For this review, take the finished solid that the model builds, in its own axes (mm). A direction names the side the tool comes from. Round coordinates to 2 decimals unless told otherwise and drop trailing zeros. Order: outer loops, then holes, each group sorted by start corner. A loop starts at its lowest first (then second) coordinate and runs counter-clockwise, first axis right, second up. Notation, with made-up numbers: M 42,7 L 65,7 A32 cw 65,43 Z; hole C 43,58.25 d5. An arc over 180 degrees is marked long. Put each result on its own line as item: value.
from build123d import *

# Parameters (mm, degrees)
F1_DEPTH = 15.24


with BuildPart() as f1:
    # F0 (on Front) → F1 (new body, symmetric)
    with BuildSketch(Plane.XZ):
        with BuildLine():
            ThreePointArc((39.819952, -34.683209), (43.15441, -51.434249), (51.5128, -66.328987))
            Line((51.5128, -66.328987), (81.9928, -66.328987))
            Line((81.9928, -66.328987), (64.616776, -18.092548))
            ThreePointArc((64.616776, -18.092548), (65.491758, -8.876663), (73.156603, -3.68549))
            Line((73.156603, -3.68549), (73.156603, 0))
            Line((73.156603, 0), (0, 0))
            Line((0, 0), (0, -7.535368))
            Line((0, -7.535368), (28.341651, -7.535368))
            Line((28.341651, -7.535368), (28.341651, -29.748611))
            Line((28.341651, -29.748611), (33.654915, -29.748611))
            ThreePointArc((33.654915, -29.748611), (37.603267, -31.134181), (39.819952, -34.683209))
        make_face()
    extrude(amount=F1_DEPTH, both=True)


solid = f1.part
(1) For faces 4 (the face through (73.157, 0, -2)), 5 (the face through (28.342, 0, -18)), 6 (the face through (73.426, -0.213, -42.548)), list the 3-axis set-ups (+Z, -Z, +X, -X, +Y, -Y) from which the entire face can be reached by the end or side of a thin tool; tool diameter is ignored.
A:
face 4: +Z, +X, +Y, -Y
face 5: -Z, -X, +Y, -Y
face 6: +X, +Y, -Y
(2) Add section A-A on x = 67. Give the boundary of the cut face in (y, z), then the cut area to 3 significant figures.
A:
outline: M -15.24,-66.33 L 15.24,-66.33 L 15.24,-24.71 L -15.24,-24.71 Z; M -15.24,-6.89 L 15.24,-6.89 L 15.24,0 L -15.24,0 Z
area: 1,480 mm2
(3) Add section B-B on y = -10. Give the boundary of the cut face in (x, z), then the cut area to 3 significant figures.
A:
outline: M 0,-7.54 L 28.34,-7.54 L 28.34,-29.75 L 33.65,-29.75 A6.32 cw 39.82,-34.68 A54.47 ccw 51.51,-66.33 L 81.99,-66.33 L 64.62,-18.09 A10.86 cw 73.16,-3.69 L 73.16,0 L 0,0 Z
area: 2,550 mm2
(4) To check wall thickness, follow L1, parallel to Z at x = 7, y = -9; L2, parallel to X at y = 9.5, z = -55.5; L3, parallel to Z at x = 32, y = -9. State the ranges of each line that lie inside material, in increasing order.
A:
L1: z = -7.54 to 0
L2: x = 44.85 to 78.09
L3: z = -29.75 to 0
(5) Draft analysis for pull direction Z (two halves, no side actions). For faces 1 (the face through (65.424, -0.213, -8.992)), 2 (the face through (67, 0, -66.329)), 3 (the face through (50, 15.24, -33)), state which applies: released by +Z, released by -Z, zero draft, split by the parting line, or undercut.
A:
face 1: undercut
face 2: released by -Z
face 3: zero draft
(6) Add section C-C on z = -47.5. Give the boundary of the cut face in (x, y), then the cut area to 3 significant figures.
A:
outline: M 41.87,-15.24 L 75.21,-15.24 L 75.21,15.24 L 41.87,15.24 Z
area: 1,020 mm2
(7) Add section D-D on x = 13. Give the boundary of the cut face in (y, z), then the cut area to 3 significant figures.
A:
outline: M -15.24,-7.54 L 15.24,-7.54 L 15.24,0 L -15.24,0 Z
area: 230 mm2
(8) Insertion check: pin 1 Ø14 at (x, y) = (11.5, -7.5) entering from -Z; pin 2 Ø1.8 at (y, z) = (5, -1) entering from +X; pin 3 Ø4.5 at (x, y) = (30, -3.5) entering from -Z. Each pin has a flat end and moves straight along its axis. Give the tip position at first contact, or say it passes through.
A:
pin 1: stops at z = -7.54
pin 2: stops at x = 73.16
pin 3: stops at z = -29.75
